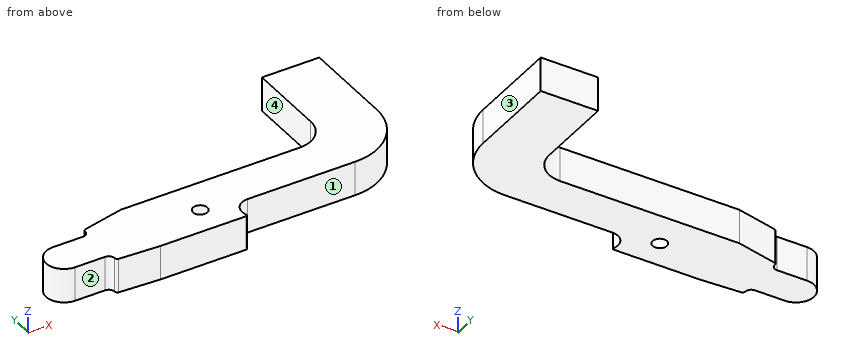
```python
from build123d import *

# Parameters (mm, degrees)
F0_R     = 1
F1_DEPTH = 4.8


with BuildPart() as f1:
    # F0 (on Top) → F1 (new body)
    with BuildSketch(Plane.XY):
        with BuildLine():
            ThreePointArc((40, 4), (45.656854, 6.343146), (48, 12))
            Line((48, 12), (48, 25))
            Line((48, 25), (40, 25))
            Line((40, 25), (40, 14))
            ThreePointArc((40, 14), (38.828427, 11.171573), (36, 10))
            Line((36, 10), (11, 10))
            Line((11, 10), (5.311352, 8.707125))
            ThreePointArc((5.311352, 8.707125), (5.087383, 8.566612), (5, 8.317072))
            Line((5, 8.317072), (5, 8.3))
            ThreePointArc((5, 8.3), (4.765685, 7.734315), (4.2, 7.5))
            Line((4.2, 7.5), (0, 7.5))
            ThreePointArc((0, 7.5), (-2.5, 5), (0, 2.5))
            Line((0, 2.5), (4.2, 2.5))
            ThreePointArc((4.2, 2.5), (4.765685, 2.265685), (5, 1.7))
            Line((5, 1.7), (5, 1.682928))
            ThreePointArc((5, 1.682928), (5.087383, 1.433388), (5.311352, 1.292875))
            Line((5.311352, 1.292875), (11, 1))
            Line((11, 1), (22.95061, 1))
            ThreePointArc((22.95061, 1), (23.115754, 1.087185), (23.136918, 1.272727))
            ThreePointArc((23.136918, 1.272727), (23.348554, 3.128152), (25, 4))
            Line((25, 4), (40, 4))
        make_face()
        with Locations((19, 5)):
            Circle(F0_R, mode=Mode.SUBTRACT)
    extrude(amount=F1_DEPTH)


solid = f1.part
```
Check sheet for the modelled part. Datum: model origin and axes. Units: mm. Face numbers are marked on the shaded views. A direction names the side the tool comes from. Round coordinates to 2 decimals unless told otherwise and drop trailing zeros. Loops run counter-clockwise (first coordinate to the right, second up) from the corner with the lowest first, then second, coordinate; pieces in that order, holes last. Notation, with made-up numbers: (-38, 52.5) -> (-26, 52.5) arc R22 cw to (-26, 85.5) -> close; hole circle Ø1 at (57, -28). An arc over 180 degrees is marked (long way). Answer in a Markdown table with one row per item.
Q1. Set-up check for the marked faces 1, 2, 3 and 4: record each of +Z, -Z, +X, -X, +Y, -Y from which the full face is reachable in a straight line by a thin tool's end or side.
Data:
| item | result |
|---|---|
| face 1 | +Z, -Z, +X, -Y |
| face 2 | +Z, -Z, -X, -Y |
| face 3 | +Z, -Z, +X, +Y, -Y |
| face 4 | +Z, -Z, -X, +Y |
Q2. Sectioned sample at C-C on y = 5. Enter the section's corners in (x, z).
Data:
| item | result |
|---|---|
| outline | (-2.5, 0) -> (18, 0) -> (18, 4.8) -> (-2.5, 4.8) -> close; (20, 0) -> (43.87, 0) -> (43.87, 4.8) -> (20, 4.8) -> close |
Q3. Go/stop test with flat-tipped pins: P1, Ø2.5, axis at x = 25, z = 2.5, coming from the +Y side; P2, Ø2, axis at y = 20, z = 3.5, coming from the -X side; P3, Ø1.6, axis at x = 19, y = 5, coming from the -Z side; P4, Ø1.5, axis at y = 7, z = 1, coming from the +X side. Record where each tip stops, or that it passes through.
Data:
| item | result |
|---|---|
| P1 | stops at y = 10 |
| P2 | stops at x = 40 |
| P3 | passes through |
| P4 | stops at x = 46.78 |
Q4. Thickness scan on L1, parallel to Y at x = 19, z = 3.25; L2, parallel to X at y = 20.75, z = 1.2; L3, parallel to Y at x = 44.5, z = 1.55. Record the ranges inside material, lowest first.
Data:
| item | result |
|---|---|
| L1 | y = 1 to 4, 6 to 10 |
| L2 | x = 40 to 48 |
| L3 | y = 5.39 to 25 |
Q5. Sectioned sample at D-D on y = 23. Enter the section's corners in (x, z).
Data:
| item | result |
|---|---|
| outline | (40, 0) -> (48, 0) -> (48, 4.8) -> (40, 4.8) -> close |
Q6. Sectioned sample at A-A on x = 19. Enter the section's corners in (y, z).
Data:
| item | result |
|---|---|
| outline | (1, 0) -> (4, 0) -> (4, 4.8) -> (1, 4.8) -> close; (6, 0) -> (10, 0) -> (10, 4.8) -> (6, 4.8) -> close |
